Check sheet for the modelled part. Datum: model origin and axes. Units: mm. A direction names the side the tool comes from. Give positions to 0.01 mm unless a question says otherwise; leave off trailing zeros. Write each loop counter-clockwise with the first axis right and the second up, starting at its lowest first coordinate (ties: lowest second). Pieces come first, ordered by that corner, then holes. Notation, with made-up numbers: (81.5, 11) -> (118.5, 11) arc R14 ccw to (118.5, 32) -> close; hole circle Ø9 at (10.5, 20.25). An arc over 180 degrees is marked (long way). Answer as a JSON object with one key per item and string values.
Autodesk Inventor part; units mm, degrees
ref_plane "YZ Plane" through (0, 0, 0) normal (1, 0, 0) x (0, 1, 0)
ref_plane "XZ Plane" through (0, 0, 0) normal (0, 1, 0) x (-1, 0, 0)
ref_plane "XY Plane" through (0, 0, 0) normal (0, 0, 1) x (1, 0, 0)
sketch "Эскиз1" plane through (0, 0, 0) normal (0, 0, 1) x (1, 0, 0)
  circle A0 centre (0, 0) radius 34
  circle A1 centre (0, 0) radius 33
  dimension "d0" = 68
  dimension "d1" = 66
extrude "Выдавливание1" add sketch "Эскиз1" along normal blind 25
sketch "Эскиз4" plane through (0, 0, 25) normal (0, 0, 1) x (1, 0, 0)
  circle A0 centre (0, 0) radius 33
extrude "Выдавливание2" add sketch "Эскиз4" against normal blind 6
sketch "Эскиз5" plane through (0, 0, 25) normal (0, 0, 1) x (1, 0, 0)
  circle A0 centre (0, 0) radius 25
  line L0 (0, 25) -> (23.7764, 7.7254)
  line L1 (23.7764, 7.7254) -> (14.6946, -20.2254)
  line L2 (14.6946, -20.2254) -> (-14.6946, -20.2254)
  line L3 (-14.6946, -20.2254) -> (-23.7764, 7.7254)
  line L4 (-23.7764, 7.7254) -> (0, 25)
  circle A1 centre (0, 0) radius 11
  line L5 (0, 25) -> (-4.9275, 9.8346)
  line L6 (0, 25) -> (4.9275, 9.8346)
  line L7 (23.7764, 7.7254) -> (7.8306, 7.7254)
  line L8 (23.7764, 7.7254) -> (10.876, -1.6473)
  line L9 (14.6946, -20.2254) -> (9.7671, -5.06)
  line L10 (14.6946, -20.2254) -> (1.7942, -10.8527)
  line L11 (-14.6946, -20.2254) -> (-1.7942, -10.8527)
  line L12 (-14.6946, -20.2254) -> (-9.7671, -5.06)
  line L13 (-7.8306, 7.7254) -> (-23.7764, 7.7254)
  line L14 (-10.876, -1.6473) -> (-23.7764, 7.7254)
  line L15 (4.9275, 9.8346) -> (9.7671, -5.06)
  line L16 (10.876, -1.6473) -> (-1.7942, -10.8527)
  line L17 (1.7942, -10.8527) -> (-10.876, -1.6473)
  line L18 (-9.7671, -5.06) -> (-4.9275, 9.8346)
  line L19 (-7.8306, 7.7254) -> (7.8306, 7.7254)
  line L20 (-7.8306, 7.7254) -> (-4.9275, 9.8346)
  line L21 (-6.3791, 8.78) -> (0, 27.7353)
  line L22 (4.9275, 9.8346) -> (7.8306, 7.7254)
  line L23 (10.876, -1.6473) -> (9.7671, -5.06)
  line L24 (1.7942, -10.8527) -> (-1.7942, -10.8527)
  line L25 (-9.7671, -5.06) -> (-10.876, -1.6473)
  line L26 (0, 27.7353) -> (6.3791, 8.78)
  line L27 (-10.3215, -3.3537) -> (-26.3778, 8.5707)
  line L28 (-26.3778, 8.5707) -> (-6.3791, 8.78)
  line L29 (0, -10.8527) -> (-16.3024, -22.4383)
  line L30 (-16.3024, -22.4383) -> (-10.3215, -3.3537)
  line L31 (10.3215, -3.3537) -> (16.3024, -22.4383)
  line L32 (16.3024, -22.4383) -> (0, -10.8527)
  line L33 (6.3791, 8.78) -> (26.3778, 8.5707)
  line L34 (26.3778, 8.5707) -> (10.3215, -3.3537)
  point P0 (23.7764, 7.7254)
  point P1 (23.7764, 7.7254)
  point P2 (-15.4339, -19.6671)
  point P3 (-10.3966, -3.5932)
  point P4 (-10.523, -3.204)
  point P5 (-24.0463, 6.8392)
  point P6 (0.2046, -10.9981)
  point P7 (-0.2046, -10.9981)
  point P8 (-13.9352, -20.756)
  point P9 (13.9352, -20.756)
  point P10 (10.523, -3.204)
  point P11 (10.3966, -3.5932)
  point P12 (15.4339, -19.6671)
  point P13 (24.0463, 6.8392)
  point P14 (23.4738, 8.6011)
  point P15 (0.9263, 24.9828)
  point P16 (6.299, 9.0179)
  point P17 (6.63, 8.7774)
  point P18 (-23.4738, 8.6011)
  point P19 (-6.63, 8.7774)
  point P20 (-6.299, 9.0179)
  point P21 (-0.9263, 24.9828)
  dimension "d8" = 22
  dimension "d7" = 50
  dimension "d15" = 360
extrude "Выдавливание3" cut sketch "Эскиз5" against normal through all contours A0 L31 L1 L34 | L1 L31 A1 L34 | L33 L0 L26 A0 | L33 A1 L26 L0 | A0 L29 L2 L32 | L2 L29 A1 L32 | L21 L4 L28 A0 | L21 A1 L28 L4 | A0 L27 L3 L30 | L3 L27 A1 L30
fillet "Сопряжение1" radius 4 10 edges at (6.299, 9.0179, 22) (6.63, 8.7774, 22) (10.523, -3.204, 22) (10.3966, -3.5932, 22) (0.2046, -10.9981, 22) (-0.2046, -10.9981, 22) (-10.523, -3.204, 22) (-10.3966, -3.5932, 22) (-6.299, 9.0179, 22) (-6.63, 8.7774, 22)
sketch "Эскиз6" plane through (0, 0, 25) normal (0, 0, 1) x (1, 0, 0)
  circle A0 centre (0, 0) radius 6
  dimension "d18" = 12
extrude "Выдавливание4" cut sketch "Эскиз6" against normal blind 5.5
sketch "Эскиз7" plane through (0, 0, 19.5) normal (0, 0, 1) x (1, 0, 0)
  circle A0 centre (0, 0) radius 2.5
  dimension "d21" = 5
extrude "Выдавливание5" add sketch "Эскиз7" along normal blind 2.5
fillet "Сопряжение2" radius 2 1 edges at (-6, 0, 19.5)
sketch "Эскиз8" plane through (0, 0, 19) normal (0, 0, -1) x (-1, 0, 0)
  circle A0 centre (0, 0) radius 4
  circle A1 centre (0, 0) radius 4.5
  dimension "d25" = 9
extrude "Выдавливание6" add sketch "Эскиз8" along normal blind 23 contours A0
sketch "Эскиз9" plane through (0, 0, -4) normal (0, 0, -1) x (-1, 0, 0)
  circle A0 centre (0, 0) radius 2.5
  dimension "d28" = 5
extrude "Выдавливание7" add sketch "Эскиз9" along normal blind 3.5
sketch "Эскиз10" plane through (0, 0, -7.5) normal (0, 0, -1) x (-1, 0, 0)
  circle A0 centre (0, 0) radius 1
  dimension "d31" = 2
extrude "Выдавливание8" cut sketch "Эскиз10" against normal blind 10
properties part number "Колесо красивое"
1. Sectioned sample at D-D, the plane x = 22. Enter the section's corners in (y, z).
Determined:
{"outline": "(-25.92, 0) -> (-24.6, 0) -> (-24.6, 19) -> (-11.87, 19) -> (-11.87, 25) -> (-25.92, 25) -> close; (5.32, 19) -> (8.62, 19) -> (8.62, 25) -> (5.32, 25) -> close; (11.87, 19) -> (24.6, 19) -> (24.6, 0) -> (25.92, 0) -> (25.92, 25) -> (11.87, 25) -> close"}
2. Access from +Z, -Z, +X, -X, +Y, -Y to the whole of each face (thin tool, end or side, straight path). Record for faces 4 (the face through (-6, 0, 23)), 5 (the face through (-11.174, -3.667, 22.042)), 6 (the face through (-2, 2, -4)), 7 (the face through (-1, -1, -7.5)).
Determined:
{"face 4": "+Z", "face 5": "+Z, -Z", "face 6": "-Z", "face 7": "-Z, +X, -X, +Y, -Y"}
3. Scan lines: L1, parallel to Y at x = -21, z = 20; L2, parallel to Y at x = 0, z = -0.75; L3, parallel to Z at x = -23.5, y = -9. Record each from-to range of solid material in increasing order. Write a range as [from, to].
Determined:
{"L1": "[-26.74, -13.56], [4.58, 8.63], [13.56, 26.74]", "L2": "[-4, -1], [1, 4]", "L3": "[19, 25]"}
4. Sectioned sample at C-C, the plane y = 20. Enter the section's corners in (x, z), plus the area to 3 significant figures.
Determined:
{"outline": "(-27.5, 0) -> (-26.25, 0) -> (-26.25, 19) -> (-15, 19) -> (-15, 25) -> (-27.5, 25) -> close; (-2.6, 19) -> (2.6, 19) -> (2.6, 25) -> (-2.6, 25) -> close; (15, 19) -> (26.25, 19) -> (26.25, 0) -> (27.5, 0) -> (27.5, 25) -> (15, 25) -> close", "area": "229 mm^2"}
5. Sectioned sample at A-A, the plane z = 7. Enter the section's corners in (x, y).
Determined:
{"outline": "circle Ø68 at (0, 0); circle Ø8 at (0, 0); hole circle Ø66 at (0, 0)"}
6. Go/stop test with flat-tipped pins: P1, Ø4, axis at x = 0, y = -1, coming from the +Z side; P2, Ø2.5, axis at x = 0, y = 0, coming from the -Z side; P3, Ø8, axis at x = -7.5, z = 17.5, coming from the -Y side; P4, Ø3, axis at x = 9, z = 13.5, coming from the +Y side. Record where each tip stops, or that it passes through.
Determined:
{"P1": "z = 22", "P2": "z = -7.5", "P3": "y = -33.82", "P4": "y = 33.16"}
7. Mould release check, pull along Y, two halves, no side actions. Record for faces 1 (the face through (7, 0, 19)), 2 (the face through (0.54, 2.44, -5.73)), 3 (the face through (7, 0, 25)): released by +Y, released by -Y, zero draft, split by the parting line, or undercut.
Determined:
{"face 1": "undercut", "face 2": "split by the parting line", "face 3": "zero draft"}
